For this review, use the dimensioned drawing (mm, ordinates from the lowest corner) and the shaded views. A direction names the side the tool comes from. Coordinates: 2 decimals unless noted, no trailing zeros. Loops run counter-clockwise (first coordinate to the right, second up) from the corner with the lowest first, then second, coordinate; pieces in that order, holes last. Notation, with made-up numbers: M 54,61 L 71,61 A26 cw 71,91 Z; hole C 80.25,44 d6. An arc over 180 degrees is marked long. Write item = value, one per line. Start each with the question number.
Q1. For the marked faces 1 and 2, list the 3-axis set-ups (+Z, -Z, +X, -X, +Y, -Y) from which the entire face can be reached by the end or side of a thin tool; tool diameter is ignored.
Q2. Clearance check with flat-ended pins moving along their axes: pin 1 Ø1.8 at (x, z) = (45.5, 12.5) entering from +Y; pin 2 Ø12 at (x, y) = (11, 11.5) entering from -Z; pin 3 Ø9 at (x, z) = (23, 12) entering from +Y. State where each tip first meets the part, or that it passes through.
Q3. We need section D-D on z = 3.75. Give the boundary of the cut face in (x, y), and give its area (3 significant figures).
Q4. We need section A-A on x = 45.5. Give the boundary of the cut face in (y, z).
Q5. Wall thickness on probe 1 along X at (y, z) = (10, 18.9); probe 2 along Y at (x, z) = (13.5, 11.25); probe 3 along Z at (x, y) = (13.5, 9.25): over which ranges is each line inside the solid? List them lowest first.
Q6. We need section B-B on y = 10. Give the boundary of the cut face in (x, z), and give its area (3 significant figures).
Q7. We need section C-C on z = 12.5. Give the boundary of the cut face in (x, y).
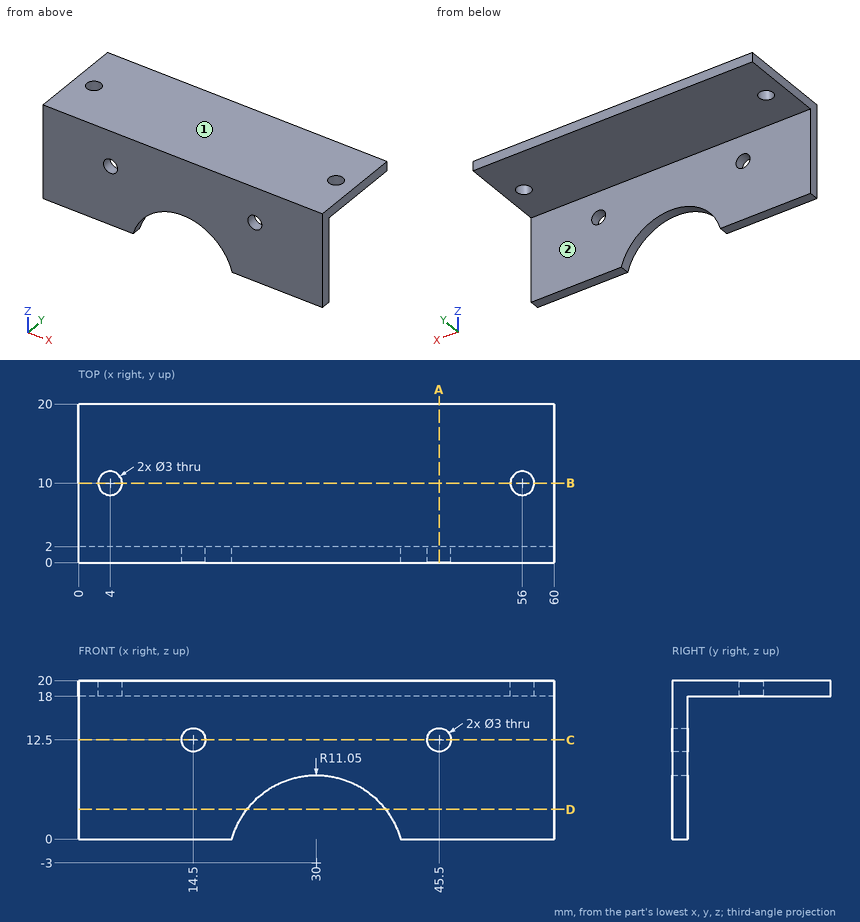
Returned:
q1.face_1 = +Z, +X, -X, +Y, -Y
q1.face_2 = -Z, +X, -X, +Y
q2.pin_1 = through
q2.pin_2 = 18
q2.pin_3 = 2
q3.outline = M 0,0 L 21.25,0 L 21.25,2 L 0,2 Z; M 38.75,0 L 60,0 L 60,2 L 38.75,2 Z
q3.area = 85.0 mm^2
q4.outline = M 0,0 L 2,0 L 2,11 L 0,11 Z; M 0,14 L 2,14 L 2,18 L 20,18 L 20,20 L 0,20 Z
q5.probe_1 = 0 to 2.5, 5.5 to 54.5, 57.5 to 60
q5.probe_2 = 0 to 2
q5.probe_3 = 18 to 20
q6.outline = M 0,18 L 2.5,18 L 2.5,20 L 0,20 Z; M 5.5,18 L 54.5,18 L 54.5,20 L 5.5,20 Z; M 57.5,18 L 60,18 L 60,20 L 57.5,20 Z
q6.area = 108 mm^2
q7.outline = M 0,0 L 13,0 L 13,2 L 0,2 Z; M 16,0 L 44,0 L 44,2 L 16,2 Z; M 47,0 L 60,0 L 60,2 L 47,2 Z
